from build123d import *

# Parameters (mm, degrees)
F0_W     = 76.2
F0_H     = 63.5
F0_W_2   = 10.9535785814
F0_H_2   = 2.4180474793
F0_H_3   = 2.414517483
F1_DEPTH = 12.7
F2_W     = 76.2
F2_H     = 13.3969295336
F3_DEPTH = 38.1
F4_R     = 3.6592600081
F4_R_2   = 3.5160030893
F5_DEPTH = 25.4


with BuildPart() as f1:
    # F0 (on Top) → F1 (new body)
    with BuildSketch(Plane.XY):
        with Locations((14.4339624465, 0.632009135)):
            Rectangle(F0_W, F0_H)
        Polygon((-10.9549575136, -9.891049689), (-10.9549575136, -16.2662230432), (-14.3190440067, -16.2662230432), (-14.3190440067, -0.1376698565), (-5.0739836443, -0.1376698565), (-5.0739836443, -2.9404869347), (-10.9549575136, -2.9404869347), (-10.9549575136, -7.0988225998), (-5.4834632174, -7.0988225998), (-5.4834632174, -9.891049689), align=None, mode=Mode.SUBTRACT)
        with Locations((2.4996234606, -10.4470241095)):
            Rectangle(F0_W_2, F0_H_2, mode=Mode.SUBTRACT)
        with Locations((2.4996234606, -6.1774935602)):
            Rectangle(F0_W_2, F0_H_3, mode=Mode.SUBTRACT)
        with BuildLine():
            Line((21.7539883888, -10.078139494), (21.7539883888, -16.2662230432))
            Line((21.7539883888, -16.2662230432), (18.3899018957, -16.2662230432))
            Line((18.3899018957, -16.2662230432), (18.3899018957, -9.0615005538))
            add(Edge.make_bspline(
                [(18.3899018957, -9.0615005538), (18.3899018957, -7.7271619448), (17.9433573612, -7.0599926403)],
                knots=[0, 0, 0, 1, 1, 1], degree=2))
            add(Edge.make_bspline(
                [(17.9433573612, -7.0599926403), (17.4968128267, -6.3928233358), (16.5366538276, -6.3928233358)],
                knots=[0, 0, 0, 1, 1, 1], degree=2))
            add(Edge.make_bspline(
                [(16.5366538276, -6.3928233358), (15.2446751745, -6.3928233358), (14.6604607835, -7.3423923459)],
                knots=[0, 0, 0, 1, 1, 1], degree=2))
            add(Edge.make_bspline(
                [(14.6604607835, -7.3423923459), (14.0762463925, -8.291961356), (14.0762463925, -10.4629090929)],
                knots=[0, 0, 0, 1, 1, 1], degree=2))
            Line((14.0762463925, -10.4629090929), (14.0762463925, -16.2662230432))
            Line((14.0762463925, -16.2662230432), (10.7121598994, -16.2662230432))
            Line((10.7121598994, -16.2662230432), (10.7121598994, -3.9324159006))
            Line((10.7121598994, -3.9324159006), (13.2819972205, -3.9324159006))
            Line((13.2819972205, -3.9324159006), (13.7338367495, -5.5103242557))
            Line((13.7338367495, -5.5103242557), (13.9209265544, -5.5103242557))
            add(Edge.make_bspline(
                [(13.9209265544, -5.5103242557), (14.4186560356, -4.6595951426), (15.3558700586, -4.1812806412)],
                knots=[0, 0, 0, 1, 1, 1], degree=2))
            add(Edge.make_bspline(
                [(15.3558700586, -4.1812806412), (16.2930840816, -3.7029661398), (17.5074028157, -3.7029661398)],
                knots=[0, 0, 0, 1, 1, 1], degree=2))
            add(Edge.make_bspline(
                [(17.5074028157, -3.7029661398), (20.2749199307, -3.7029661398), (21.259788904, -5.5103242557)],
                knots=[0, 0, 0, 1, 1, 1], degree=2))
            Line((21.259788904, -5.5103242557), (21.5563085949, -5.5103242557))
            add(Edge.make_bspline(
                [(21.5563085949, -5.5103242557), (22.054038076, -4.6490051536), (23.0177270714, -4.1759856467)],
                knots=[0, 0, 0, 1, 1, 1], degree=2))
            add(Edge.make_bspline(
                [(23.0177270714, -4.1759856467), (23.9814160668, -3.7029661398), (25.1957348009, -3.7029661398)],
                knots=[0, 0, 0, 1, 1, 1], degree=2))
            add(Edge.make_bspline(
                [(25.1957348009, -3.7029661398), (27.2925526151, -3.7029661398), (28.3674364946, -4.7778500193)],
                knots=[0, 0, 0, 1, 1, 1], degree=2))
            add(Edge.make_bspline(
                [(28.3674364946, -4.7778500193), (29.4423203741, -5.8527338988), (29.4423203741, -8.2248914259)],
                knots=[0, 0, 0, 1, 1, 1], degree=2))
            Line((29.4423203741, -8.2248914259), (29.4423203741, -16.2662230432))
            Line((29.4423203741, -16.2662230432), (26.067643892, -16.2662230432))
            Line((26.067643892, -16.2662230432), (26.067643892, -9.0615005538))
            add(Edge.make_bspline(
                [(26.067643892, -9.0615005538), (26.067643892, -7.7271619448), (25.6210993575, -7.0599926403)],
                knots=[0, 0, 0, 1, 1, 1], degree=2))
            add(Edge.make_bspline(
                [(25.6210993575, -7.0599926403), (25.174554823, -6.3928233358), (24.2143958239, -6.3928233358)],
                knots=[0, 0, 0, 1, 1, 1], degree=2))
            add(Edge.make_bspline(
                [(24.2143958239, -6.3928233358), (22.9788971119, -6.3928233358), (22.3664427504, -7.2753224158)],
                knots=[0, 0, 0, 1, 1, 1], degree=2))
            add(Edge.make_bspline(
                [(22.3664427504, -7.2753224158), (21.7539883888, -8.1578214958), (21.7539883888, -10.078139494)],
                knots=[0, 0, 0, 1, 1, 1], degree=2))
        make_face(mode=Mode.SUBTRACT)
        with BuildLine():
            Line((43.0751661625, -16.2662230432), (40.7277186096, -16.2662230432))
            Line((40.7277186096, -16.2662230432), (40.0746692903, -14.5894747911))
            Line((40.0746692903, -14.5894747911), (39.9864193823, -14.5894747911))
            add(Edge.make_bspline(
                [(39.9864193823, -14.5894747911), (39.1392202655, -15.6590636761), (38.2390712039, -16.0738382438)],
                knots=[0, 0, 0, 1, 1, 1], degree=2))
            add(Edge.make_bspline(
                [(38.2390712039, -16.0738382438), (37.3389221422, -16.4886128114), (35.8951536473, -16.4886128114)],
                knots=[0, 0, 0, 1, 1, 1], degree=2))
            add(Edge.make_bspline(
                [(35.8951536473, -16.4886128114), (34.1195654983, -16.4886128114), (33.0993965617, -15.4719738712)],
                knots=[0, 0, 0, 1, 1, 1], degree=2))
            add(Edge.make_bspline(
                [(33.0993965617, -15.4719738712), (32.0792276252, -14.455334931), (32.0792276252, -12.580906885)],
                knots=[0, 0, 0, 1, 1, 1], degree=2))
            add(Edge.make_bspline(
                [(32.0792276252, -12.580906885), (32.0792276252, -10.618228931), (33.4523961938, -9.6863099025)],
                knots=[0, 0, 0, 1, 1, 1], degree=2))
            add(Edge.make_bspline(
                [(33.4523961938, -9.6863099025), (34.8255647623, -8.7543908739), (37.5930818773, -8.655550977)],
                knots=[0, 0, 0, 1, 1, 1], degree=2))
            Line((37.5930818773, -8.655550977), (39.7357896436, -8.5884810469))
            Line((39.7357896436, -8.5884810469), (39.7357896436, -8.0483916099))
            add(Edge.make_bspline(
                [(39.7357896436, -8.0483916099), (39.7357896436, -6.1739635639), (37.8154716454, -6.1739635639)],
                knots=[0, 0, 0, 1, 1, 1], degree=2))
            add(Edge.make_bspline(
                [(37.8154716454, -6.1739635639), (36.3364031873, -6.1739635639), (34.3384252701, -7.0670526329)],
                knots=[0, 0, 0, 1, 1, 1], degree=2))
            Line((34.3384252701, -7.0670526329), (33.2264764293, -4.7937350027))
            add(Edge.make_bspline(
                [(33.2264764293, -4.7937350027), (35.3550642103, -3.6782561656), (37.9460815093, -3.6782561656)],
                knots=[0, 0, 0, 1, 1, 1], degree=2))
            add(Edge.make_bspline(
                [(37.9460815093, -3.6782561656), (40.4276689223, -3.6782561656), (41.7514175424, -4.7602000377)],
                knots=[0, 0, 0, 1, 1, 1], degree=2))
            add(Edge.make_bspline(
                [(41.7514175424, -4.7602000377), (43.0751661625, -5.8421439098), (43.0751661625, -8.0483916099)],
                knots=[0, 0, 0, 1, 1, 1], degree=2))
            Line((43.0751661625, -8.0483916099), (43.0751661625, -16.2662230432))
        make_face(mode=Mode.SUBTRACT)
    extrude(amount=F1_DEPTH)

    # F2 (on face) → F3 (join)
    with BuildSketch(Plane.XY.offset(12.7)):
        with Locations((14.4339624465, 25.6835443682)):
            Rectangle(F2_W, F2_H)
    extrude(amount=F3_DEPTH)

    # F4 (on face) → F5 (join)
    with BuildSketch(Plane(origin=(0, 0, 0), x_dir=(1, 0, 0), z_dir=(0, 0, -1))):
        with Locations((46.7344261706, -25.6791654974)):
            Circle(F4_R)
        with Locations((46.7344261706, 25.3488849849)):
            Circle(F4_R)
        with Locations((-17.835047096, -25.6791654974)):
            Circle(F4_R_2)
        with Locations((-17.835047096, 25.3488849849)):
            Circle(F4_R_2)
    extrude(amount=F5_DEPTH)


solid = f1.part
Source: CAD feature listing. Evaluate the final solid. Frame: model axes, mm. A direction names the side the tool comes from. Round coordinates to 2 decimals unless told otherwise and drop trailing zeros. Write each loop counter-clockwise with the first axis right and the second up, starting at its lowest first coordinate (ties: lowest second). Pieces come first, ordered by that corner, then holes. Notation, with made-up numbers: M 54.25,28 L 100.25,28 A19 ccw 100.25,54 Z; hole C 11.5,76 d10. An arc over 180 degrees is marked long. One line per item, written item: value. Start each with the question number.
Item 1: Section query C-C (z = -16.5). Return the cut outline in (x, y), plus the area to 3 significant figures.
Item 2: Section query B-B (x = 12). Return the cut outline in (y, z).
Item 3: Section query A-A (x = -1.5). Return the cut outline in (y, z), plus the area to 3 significant figures.
Item 4: Set-up query: faces 4 (the flat face through (14, 1, 0)), 5 (the flat face through (-10.955, -13, 6)), 6 (the flat face through (14, 18.985, 31)). Return all of +Z, -Z, +X, -X, +Y, -Y with unobstructed straight access to the full face (end or side cutting, diameter ignored); none if empty.
Item 5: Pin query (flat end, axial travel): pin 1 (2 mm diameter, centred on x = 44, z = 31, fed in from -Y); pin 2 (1.5 mm diameter, centred on y = 21, z = -1.5, fed in from +X); pin 3 (15 mm diameter, centred on x = 21.5, y = -14.5, fed in from +Z); pin 4 (2 mm diameter, centred on x = 1.5, y = 13.5, fed in from -Z). Return the tip coordinate at first contact, or that it passes through.
Item 6: Ray query, L1, parallel to Y at x = 33.5, z = 3.5; L2, parallel to Z at x = 41.5, y = 11; L3, parallel to Z at x = 19.5, y = 21. Return the intervals inside material, ascending. Write a range as from..to.
Item 7: Section query D-D (x = -13). Return the cut outline in (y, z), plus the area to 3 significant figures.
Item 8: Mould query, pull axis X, two halves, no side actions, for faces 1 (the flat face through (-23.666, 14, 8)), 2 (the flat face through (52.534, 14, 8)), 3 (the cylindrical face through (-15.94, -28.31, -12.52)). Classes: pulls with the +X half, pulls with the -X half, needs draft (parallel to the pull), parting line crosses it, or undercut.
Result set:
1. outline: C -17.84,-25.35 d7.03; C -17.84,25.68 d7.03; C 46.73,-25.35 d7.32; C 46.73,25.68 d7.32
1. area: 162 mm²
2. outline: M -31.12,0 L -16.27,0 L -16.27,12.7 L -31.12,12.7 Z; M -3.93,0 L 32.38,0 L 32.38,50.8 L 18.99,50.8 L 18.99,12.7 L -3.93,12.7 Z
3. outline: M -31.12,0 L -11.66,0 L -11.66,12.7 L -31.12,12.7 Z; M -9.24,0 L -7.38,0 L -7.38,12.7 L -9.24,12.7 Z; M -4.97,0 L 32.38,0 L 32.38,50.8 L 18.99,50.8 L 18.99,12.7 L -4.97,12.7 Z
3. area: 1,260 mm²
4. face 4: -Z
4. face 5: +Z, -Z
4. face 6: +Z, +X, -X, -Y
5. pin 1: stops at y = 18.99
5. pin 2: passes through
5. pin 3: stops at z = 12.7
5. pin 4: stops at z = 0
6. L1: y = -31.12..-15.81, -9.65..-5.35, -4.66..32.38
6. L2: z = 0..12.7
6. L3: z = 0..50.8
7. outline: M -31.12,0 L -16.27,0 L -16.27,12.7 L -31.12,12.7 Z; M -0.14,0 L 32.38,0 L 32.38,50.8 L 18.99,50.8 L 18.99,12.7 L -0.14,12.7 Z
7. area: 1,110 mm²
8. face 1: pulls with the -X half
8. face 2: pulls with the +X half
8. face 3: undercut
